Part model, mm, in its own coordinate system. Face numbers are marked on the shaded views. A direction names the side the tool comes from. Round coordinates to 2 decimals unless told otherwise and drop trailing zeros. Write each loop counter-clockwise with the first axis right and the second up, starting at its lowest first coordinate (ties: lowest second). Pieces come first, ordered by that corner, then holes.
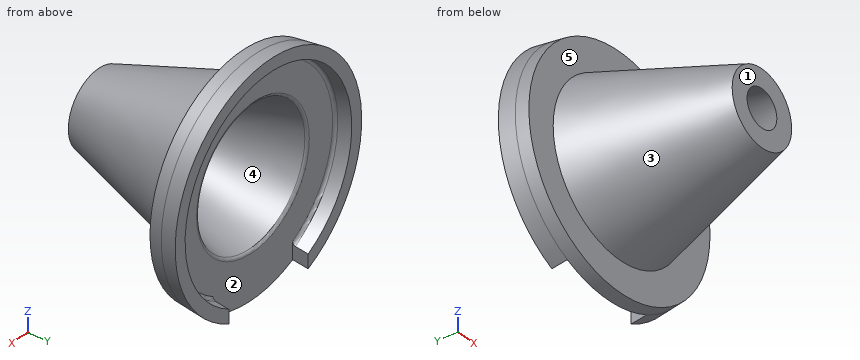
from build123d import *

# Parameters (mm, degrees)
SKETCH2_W          = 32
SKETCH2_H          = 5
CUT_EXTRUDE2_DEPTH = 77.50062169
FILLET1_R          = 1
FILLET2_R          = 1


with BuildPart() as part:
    # Sketch1 → Revolve1 (revolve)
    with BuildSketch(Plane.XY):
        Polygon((-12, 0), (-6, 0), (-22, 50), (-22, 46), (-26.72, 46), align=None)
        Polygon((-36.520930233, 46), (-26.72, 46), (-28, 50), (-33, 50), (-37, 50), align=None)
        Polygon((-22, 46), (-22, 50), (-28, 50), (-26.72, 46), align=None)
        Polygon((-37, 50), (-33, 50), (-33.598837209, 55), (-37.598837209, 55), align=None)
    revolve(axis=Axis((0, 50, 0), (0, -1, 0)))

    # Sketch2 → Cut-Extrude2 (cut, through all)
    with BuildSketch(Plane.XY):
        with Locations((0, 52.5)):
            Rectangle(SKETCH2_W, SKETCH2_H)
    extrude(amount=-CUT_EXTRUDE2_DEPTH, mode=Mode.SUBTRACT)

    # Fillet1
    fillet1_edges = [part.edges().sort_by_distance(p)[0] for p in [
        (0, 50, 33),
    ]]
    fillet(fillet1_edges, radius=FILLET1_R)

    # Fillet2
    fillet2_edges = [part.edges().sort_by_distance(p)[0] for p in [
        (22, 50, 0),
    ]]
    fillet(fillet2_edges, radius=FILLET2_R)


solid = part.part
Q1. Saw through at B-B, the plane y = 35. Write the cut outline in (x, z).
Q2. Two-plate mould, pull along Z, no slides. Class the marked faces 1, 2 and 3: released by +Z, released by -Z, zero draft, split by the parting line, or undercut.
Q3. Wall check: line 1 (X direction, y = 25.5, z = -11.5); line 2 (Y direction, x = -17, z = 24); line 3 (Z direction, x = 11, y = 30.5). Give the ranges that are in metal, low to high.
Q4. Saw through at A-A, the plane y = 15. Write the cut outline in (x, z).
Q5. Tool access for the marked faces 4 and 5: list every direction of +Z, -Z, +X, -X, +Y, -Y with a clear straight run to the whole face (end or side of a thin tool).
Q6. Drop flat-ended pins along their axis: P1, Ø1.5, axis at x = 27.5, z = -1.5, coming from the +Y side; P2, Ø3, axis at y = 26, z = -11, coming from the -X side; P3, Ø5, axis at y = 37, z = 0, coming from the +X side. Give the stop position or say it passes through.
Computed:
1. outline: circle Ø46.4 at (0, 0); hole circle Ø34.4 at (0, 0)
2. face 1: zero draft
2. face 2: undercut
2. face 3: split by the parting line
3. line 1: x = -16.56 to -8.26, 8.26 to 16.56
3. line 2: y = 46 to 50
3. line 3: z = -18.77 to -11.29, 11.29 to 18.77
4. outline: circle Ø33.6 at (0, 0); hole circle Ø21.6 at (0, 0)
5. face 4: +Y
5. face 5: -Y
6. P1: stops at y = 50
6. P2: stops at x = -18.13
6. P3: stops at x = 24.64
